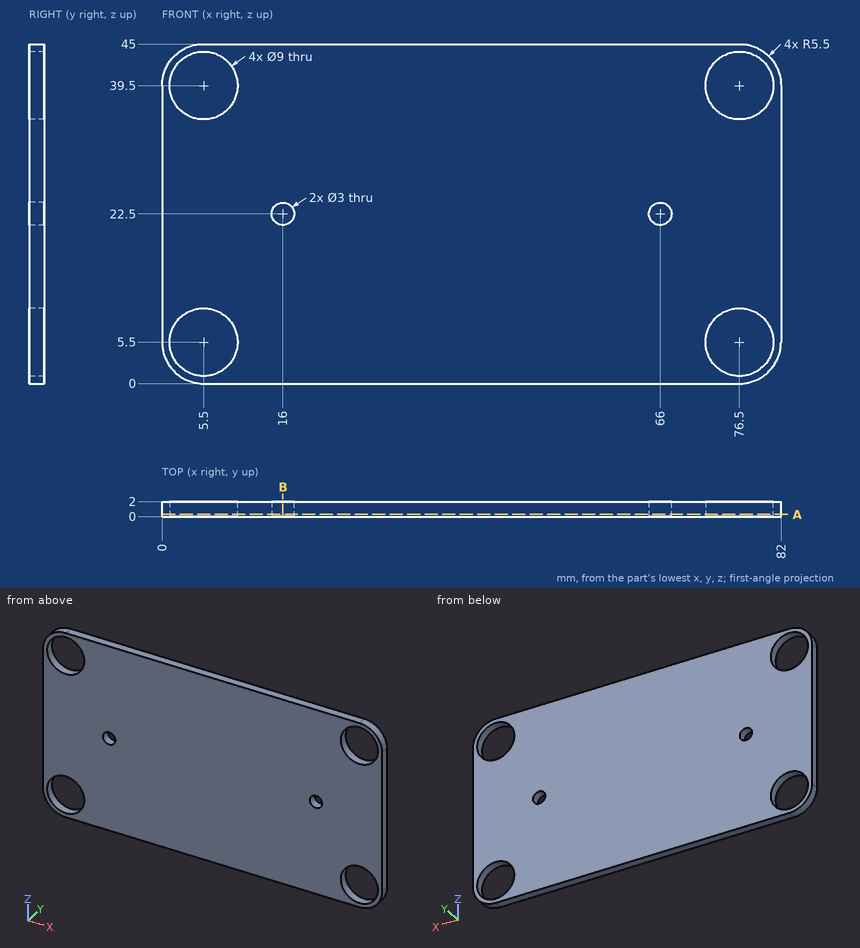
Geometry check sheet. Reference: drawing and pictorial views, mm from the part's lowest x, y, z. Round coordinates to 2 decimals unless told otherwise and drop trailing zeros. Loops run counter-clockwise (first coordinate to the right, second up) from the corner with the lowest first, then second, coordinate; pieces in that order, holes last. Notation, with made-up numbers: (60.5, 39.5) - (109.5, 39.5) arc R29 cw to (109.5, 73.5) - close; hole circle Ø5 at (84, -23.5). An arc over 180 degrees is marked (long way). Answer in a Markdown table with one row per item. Add a question column.
Q1. Gauge pin test, flat end, axial feed: pin 1 (2.5 mm diameter, centred on x = 66, z = 22.5, fed in from -Y). Record the tip position at first contact, or that the pin passes through.
Q2. Section check B-B on x = 16. Enter the section's corners in (y, z).
Q3. Material ranges on line 1 (X direction, y = 1.25, z = 22.5); line 2 (Z direction, x = 76.5, y = 1.4); line 3 (X direction, y = 1, z = 39.5), recorded low to high.
Q4. Section check A-A on y = 0.3. Enter the section's corners in (x, z), plus the area to 3 significant figures.
Found:
| question | item | result |
|---|---|---|
| 1 | pin 1 | passes through |
| 2 | outline | (0, 0) - (2, 0) - (2, 21) - (0, 21) - close; (0, 24) - (2, 24) - (2, 45) - (0, 45) - close |
| 3 | line 1 | x = 0 to 14.5, 17.5 to 64.5, 67.5 to 82 |
| 3 | line 2 | z = 0 to 1, 10 to 35, 44 to 45 |
| 3 | line 3 | x = 0 to 1, 10 to 72, 81 to 82 |
| 4 | outline | (0, 5.5) arc R5.5 ccw to (5.5, 0) - (76.5, 0) arc R5.5 ccw to (82, 5.5) - (82, 39.5) arc R5.5 ccw to (76.5, 45) - (5.5, 45) arc R5.5 ccw to (0, 39.5) - close; hole circle Ø9 at (5.5, 5.5); hole circle Ø9 at (5.5, 39.5); hole circle Ø3 at (16, 22.5); hole circle Ø3 at (66, 22.5); hole circle Ø9 at (76.5, 5.5); hole circle Ø9 at (76.5, 39.5) |
| 4 | area | 3,400 mm² |
